from build123d import *

# Parameters (mm, degrees)
BOSS_EXTRUDE2_DEPTH             = 38
BOSS_EXTRUDE2_DEPTH_BACK        = 38
FILLET1_R                       = 30
CUT_EXTRUDE1_DEPTH              = 111.453610172
CUT_EXTRUDE1_DEPTH_BACK         = 111.453610172
SKETCH3_R                       = 15
BOSS_EXTRUDE3_REACH             = 112.454
SKETCH5_W                       = 100
SKETCH5_H                       = 12
BOSS_EXTRUDE3_DIRECTION_2_REACH = 112.454
RIB1_REACH                      = 117.135
SKETCH7_WALL_W                  = 362.269405062
SKETCH7_WALL_H                  = 10


with BuildPart() as part:
    # Sketch2 → Boss-Extrude2 (new, two sides: drawn at the far end of the back side and taken through both)
    with BuildSketch(Plane(origin=(0, 0, 0), x_dir=(0, 0, -1), z_dir=(1, 0, 0)).offset(-BOSS_EXTRUDE2_DEPTH_BACK)):
        Polygon((-80, 6), (20, 6), (20, 66), (80, 66), (80, 6), (80, -6), (-80, -6), align=None)
    extrude(amount=BOSS_EXTRUDE2_DEPTH + BOSS_EXTRUDE2_DEPTH_BACK)

    # Fillet1
    fillet1_edges = [part.edges().sort_by_distance(p)[0] for p in [
        (0, 66, -80),
        (0, 66, -20),
    ]]
    fillet(fillet1_edges, radius=FILLET1_R - 0.0001)  # a hair under: the kernel refuses the full size

    # Sketch3 → Cut-Extrude1 (cut, two sides: drawn at the far end of the back side and taken through both)
    with BuildSketch(Plane(origin=(0, 0, 0), x_dir=(0, 0, -1), z_dir=(1, 0, 0)).offset(-CUT_EXTRUDE1_DEPTH_BACK)):
        with Locations((50, 36)):
            Circle(SKETCH3_R)
    extrude(amount=CUT_EXTRUDE1_DEPTH + CUT_EXTRUDE1_DEPTH_BACK, mode=Mode.SUBTRACT)

    # Boss-Extrude3: up to this face of the body (flat: up to its plane)
    boss_extrude3_end = Plane(part.part.faces().sort_by_distance((0, 0, 80))[0])
    # Sketch5 → Boss-Extrude3 (add, up to the picked face)
    with BuildSketch(Plane.XY, mode=Mode.PRIVATE) as boss_extrude3_sk1:
        with Locations((0, -12)):
            Rectangle(SKETCH5_W, SKETCH5_H)
    boss_extrude3_tool1 = split(extrude(boss_extrude3_sk1.sketch, amount=BOSS_EXTRUDE3_REACH, mode=Mode.PRIVATE), bisect_by=boss_extrude3_end, keep=Keep.BOTH, mode=Mode.PRIVATE)
    add(boss_extrude3_tool1.solids().sort_by(Axis((0, -12, 0), (0, 0, 1)))[0])

    # Boss-Extrude3 direction 2: up to this face of the body (flat: up to its plane)
    boss_extrude3_direction_2_end = Plane(part.part.faces().sort_by_distance((0, 15.00005, -80))[0])
    # Sketch5 → Boss-Extrude3 direction 2 (add, up to the picked face)
    with BuildSketch(Plane.XY, mode=Mode.PRIVATE) as boss_extrude3_direction_2_sk1:
        with Locations((0, -12)):
            Rectangle(SKETCH5_W, SKETCH5_H)
    boss_extrude3_direction_2_tool1 = split(extrude(boss_extrude3_direction_2_sk1.sketch, amount=-BOSS_EXTRUDE3_DIRECTION_2_REACH, mode=Mode.PRIVATE), bisect_by=boss_extrude3_direction_2_end, keep=Keep.BOTH, mode=Mode.PRIVATE)
    add(boss_extrude3_direction_2_tool1.solids().sort_by(Axis((0, -12, 0), (0, 0, -1)))[0])

    # Sketch7 wall → Rib1 (add, up to next)
    with BuildSketch(Plane(origin=(0, 34.483145548, 21.573034774), x_dir=(0, 0.438202247192, -0.898876404494), z_dir=(0, 0.898876404494, 0.438202247192)), mode=Mode.PRIVATE) as rib1_sk1:
        Rectangle(SKETCH7_WALL_W, SKETCH7_WALL_H)
    rib1_tool1 = extrude(rib1_sk1.sketch, amount=-RIB1_REACH, mode=Mode.PRIVATE) - part.part
    add(rib1_tool1.solids().sort_by_distance((0, 34.483145548, 21.573034774))[0])


solid = part.part
Geometry check sheet. Reference: the model listing, model coordinates, mm. A direction names the side the tool comes from. Give positions to 0.01 mm unless a question says otherwise; leave off trailing zeros. Order: outer loops, then holes, each group sorted by start corner. A loop starts at its lowest first (then second) coordinate and runs counter-clockwise, first axis right, second up. Notation, with made-up numbers: (14, -32) - (53, -32) arc R22 cw to (53, 1) - close; hole circle Ø11 at (-25, 23). An arc over 180 degrees is marked (long way). Answer as a JSON object with one key per item and string values.
(1) Cross-section at B-B (z = -46). Record the cut outline in (x, y).
Report:
{"outline": "(-50, -18) - (50, -18) - (50, -6) - (38, -6) - (38, 21.54) - (-38, 21.54) - (-38, -6) - (-50, -6) - close; (-38, 50.46) - (38, 50.46) - (38, 65.73) - (-38, 65.73) - close"}
(2) Cross-section at D-D (y = 15). Record the cut outline in (x, z).
Report:
{"outline": "(-38, -80) - (38, -80) - (38, -20) - (5, -20) - (5, 61.54) - (-5, 61.54) - (-5, -20) - (-38, -20) - close"}
(3) Depth check by flat-ended pin: pin 1 Ø10 at (x, z) = (28.5, 10) entering from +Y; pin 2 Ø6 at (x, z) = (-42, -21) entering from +Y; pin 3 Ø4 at (x, y) = (12, 50) entering from -Z. Enter the tip coordinate at first touch or a pass-through.
Report:
{"pin 1": "y = 6", "pin 2": "y = -6", "pin 3": "z = -77.5"}
(4) Draft check along Y on faces 4 (the flat face through (-22, 6, 31)), 5 (the flat face through (-1, -6, 80)), 6 (the flat face through (-1, -18, 1)), 7 (the cylindrical face through (-0.532, 46.138, -38.944)). Enter one of: released by +Y, released by -Y, zero draft, split by the parting line, or undercut.
Report:
{"face 4": "released by +Y", "face 5": "zero draft", "face 6": "released by -Y", "face 7": "undercut"}
(5) Cross-section at C-C (z = 32). Record the cut outline in (x, y), then the cut area to 3 significant figures.
Report:
{"outline": "(-50, -18) - (50, -18) - (50, -6) - (38, -6) - (38, 6) - (5, 6) - (5, 29.4) - (-5, 29.4) - (-5, 6) - (-38, 6) - (-38, -6) - (-50, -6) - close", "area": "2,350 mm^2"}
(6) Material ranges on line 1 (Y direction, x = 17.5, z = -50); line 2 (X direction, y = 59, z = -59); line 3 (Y direction, x = -31, z = 4), recorded low to high.
Report:
{"line 1": "-18 to 21, 51 to 66", "line 2": "-38 to 38", "line 3": "-18 to 6"}
(7) Tool access check on faces 1 (the flat face through (21, 6, 31)), 2 (the flat face through (-5, 23, 17)), 3 (the flat face through (44, -6, 1)). Record the directions out of +Z, -Z, +X, -X, +Y, -Y that give a thin tool (end or side, any length) a straight path to the whole face; none if there is none.
Report:
{"face 1": "+Z, +X, +Y", "face 2": "+Z, -X, +Y", "face 3": "+Z, -Z, +X, +Y"}
